```python
from build123d import *

# Parameters (mm, degrees)
SKETCH1_W           = 28
SKETCH1_H           = 57
BOSS_EXTRUDE1_DEPTH = 5
BOSS_EXTRUDE2_DEPTH = 6
SKETCH3_R           = 2.25
CUT_EXTRUDE1_DEPTH  = 60.715994507
SKETCH4_R           = 2.25
CUT_EXTRUDE2_DEPTH  = 60
SKETCH5_R           = 8
BOSS_EXTRUDE3_DEPTH = 7.5
SKETCH6_R           = 2.25
CUT_EXTRUDE3_DEPTH  = 61.010415763


with BuildPart() as part:
    # Sketch1 → Boss-Extrude1 (new body)
    with BuildSketch(Plane.XY):
        with Locations((0, -28.5)):
            Rectangle(SKETCH1_W, SKETCH1_H)
    extrude(amount=BOSS_EXTRUDE1_DEPTH)

    # Sketch2 → Boss-Extrude2 (add, symmetric)
    with BuildSketch(Plane(origin=(0, 0, 0), x_dir=(0, 0, -1), z_dir=(1, 0, 0))):
        with BuildLine():
            Line((-5, 0), (-5, -24))
            Line((-5, -24), (-11, -24))
            Line((-11, -24), (-11, -16))
            ThreePointArc((-11, -16), (-7, -12), (-11, -8))
            Line((-11, -8), (-11, 0))
            Line((-11, 0), (-5, 0))
        make_face()
    extrude(amount=BOSS_EXTRUDE2_DEPTH, both=True)

    # Sketch3 → Cut-Extrude1 (cut, through all)
    with BuildSketch(Plane.XY.offset(11)):
        with Locations((0, -4)):
            Circle(SKETCH3_R)
        with Locations((0, -20)):
            Circle(SKETCH3_R)
    extrude(amount=-CUT_EXTRUDE1_DEPTH, mode=Mode.SUBTRACT)

    # Sketch4 → Cut-Extrude2 (cut, through all)
    with BuildSketch(Plane.XY.offset(5)):
        with Locations((-9, -51)):
            Circle(SKETCH4_R)
        with Locations((9, -51)):
            Circle(SKETCH4_R)
    extrude(amount=-CUT_EXTRUDE2_DEPTH, mode=Mode.SUBTRACT)

    # Sketch5 → Boss-Extrude3 (add)
    with BuildSketch(Plane.XY.offset(5)):
        with Locations((0, -36)):
            Circle(SKETCH5_R)
    extrude(amount=BOSS_EXTRUDE3_DEPTH)

    # Sketch6 → Cut-Extrude3 (cut, through all)
    with BuildSketch(Plane.XY.offset(12.5)):
        with Locations((0, -36)):
            Circle(SKETCH6_R)
    extrude(amount=-CUT_EXTRUDE3_DEPTH, mode=Mode.SUBTRACT)


solid = part.part
```
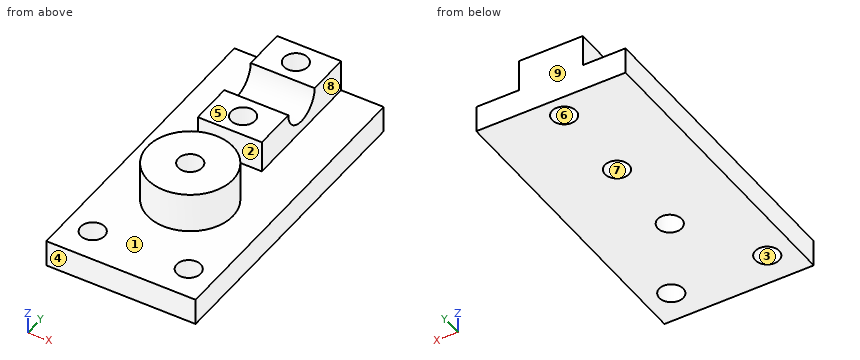
Verification items for the finished model (mm, model axes). Face numbers are marked on the shaded views. A direction names the side the tool comes from. Round coordinates to 2 decimals unless told otherwise and drop trailing zeros. Write each loop counter-clockwise with the first axis right and the second up, starting at its lowest first coordinate (ties: lowest second). Pieces come first, ordered by that corner, then holes.
1. Draft check along Y on the marked faces 6, 7, 8 and 9. Enter one of: +Y half, -Y half, draft (parallel to the pull), parting line (faces both ways), or undercut.
2. Section check B-B on y = -20. Enter the section's corners in (x, z), plus the area to 4 significant figures.
3. Section check A-A on z = 3. Enter the section's corners in (x, y), plus the area to 3 significant figures.
4. Scan lines: L1, parallel to Y at x = 9, z = 3.85; L2, parallel to Z at x = 0, y = -53.5; L3, parallel to Z at x = -5, y = -17.5. Record each from-to range of solid material in increasing order.
5. Access from +Z, -Z, +X, -X, +Y, -Y to the whole of each face (thin tool, end or side, straight path). Record for the marked faces 1, 2, 3, 4 and 5.
6. Section check C-C on x = 9. Enter the section's corners in (y, z), plus the area to 4 significant figures.
7. Gauge pin test, flat ends, axial feed: P1, Ø7, axis at x = -9, y = -51, coming from the -Z side; P2, Ø6, axis at x = 9, y = -51, coming from the +Z side; P3, Ø9, axis at x = 2, y = -2.5, coming from the +Z side; P4, Ø3, axis at y = -9.5, z = 8.5, coming from the -X side. Record the tip position at first contact, or that the pin passes through.
8. Section check D-D on z = 8.5. Enter the section's corners in (x, y), plus the area to 3 significant figures.
Answer:
1. face 6: undercut
1. face 7: undercut
1. face 8: draft
1. face 9: +Y half
2. outline: (-14, 0) - (-2.25, 0) - (-2.25, 11) - (-6, 11) - (-6, 5) - (-14, 5) - close; (2.25, 0) - (14, 0) - (14, 5) - (6, 5) - (6, 11) - (2.25, 11) - close
2. area: 162.5 mm2
3. outline: (-14, -57) - (14, -57) - (14, 0) - (-14, 0) - close; hole circle Ø4.5 at (-9, -51); hole circle Ø4.5 at (0, -36); hole circle Ø4.5 at (0, -20); hole circle Ø4.5 at (0, -4); hole circle Ø4.5 at (9, -51)
3. area: 1,520 mm2
4. L1: y = -57 to -53.25, -48.75 to 0
4. L2: z = 0 to 5
4. L3: z = 0 to 11
5. face 1: +Z
5. face 2: +Z, +X, -X
5. face 3: +Z, -Z
5. face 4: +Z, -Z, +X, -X, -Y
5. face 5: +Z, +X, -X, +Y
6. outline: (-57, 0) - (-53.25, 0) - (-53.25, 5) - (-57, 5) - close; (-48.75, 0) - (0, 0) - (0, 5) - (-48.75, 5) - close
6. area: 262.5 mm2
7. P1: stops at z = 0
7. P2: stops at z = 5
7. P3: stops at z = 11
7. P4: stops at x = -6
8. outline: circle Ø16 at (0, -36); (-6, -24) - (6, -24) - (6, -15.12) - (-6, -15.12) - close; (-6, -8.88) - (6, -8.88) - (6, 0) - (-6, 0) - close; hole circle Ø4.5 at (0, -36); hole circle Ø4.5 at (0, -20); hole circle Ø4.5 at (0, -4)
8. area: 366 mm2
